Autodesk Inventor part; units mm, degrees
ref_plane "YZ Plane" through (0, 0, 0) normal (1, 0, 0) x (0, 1, 0)
ref_plane "XZ Plane" through (0, 0, 0) normal (0, 1, 0) x (-1, 0, 0)
ref_plane "XY Plane" through (0, 0, 0) normal (0, 0, 1) x (1, 0, 0)
sketch "Sketch1" plane through (0, 0, 0) normal (0, 0, 1) x (1, 0, 0)
  line L0 (0, 0) -> (50, 0)
  line L1 (50, 0) -> (140.0002, 119.9998)
  line L2 (140.0002, 119.9998) -> (141.8074, 169.9998)
  line L3 (172.7872, 168.8801) -> (170.5233, 106.2458)
  line L4 (0, -10) -> (50, -10)
  arc A0 (50, -10) -> (170.5233, 106.2458) centre (50, 110.602) ccw
  line L5 (0, -10) -> (0, 0)
  line L6 (141.8074, 169.9998) -> (172.7872, 168.8801)
  line L7 (140.0002, 119.9998) -> (171.0205, 119.9998)
  dimension "d0" = 150
  dimension "d1" = 126.87
  dimension "d2" = 50
  dimension "d3" = 145.2
  dimension "d4" = 31
  dimension "d5" = 10
  dimension "d6" = 50
extrude "Extrusion1" add sketch "Sketch1" along normal blind 25
sketch "Sketch2" plane through (0, -10, 0) normal (0, -1, 0) x (1, 0, 0)
  line L0 (0, 0) -> (50, 0)
  line L1 (50, 0) -> (50, 25)
  line L2 (0, 25) -> (50, 25)
  line L3 (0, 0) -> (0, 25)
  circle A0 centre (25, 12.5) radius 1.65
  point P0 (50, 12.5)
  point P1 (25, 25)
  dimension "d9" = 3.3
extrude "Extrusion2" cut sketch "Sketch2" against normal through all contours A0
sketch "Sketch3" plane through (172.7872, 168.8801, 25) normal (0.9993, -0.0361, 0) x (0, 0, -1)
  line L0 (25, -62.6752) -> (25, 0)
  line L1 (25, 0) -> (0, 0)
  line L2 (0, -62.6752) -> (0, 0)
  line L3 (25, -62.6752) -> (0, -62.6752)
  circle A0 centre (12.5, -22.6752) radius 2.15
  point P0 (25, -175.0111)
  point P1 (12.5, -62.6752)
  dimension "d12" = 4.3
  dimension "d13" = 40
extrude "Extrusion3" cut sketch "Sketch3" against normal through all contours A0
chamfer "Chamfer1" distance 10 angle 45 1 edges at (141.8074, 169.9998, 12.5)
properties part number "ESQUINA_REDONDEADA_TRASERA" material "Steel, Mild, Welded"
Input: part model. Units: mm. Frame: model coordinates. Give positions to 0.01 mm unless a question says otherwise; leave off trailing zeros. Order: outer loops, then holes, each group sorted by start corner. A loop starts at its lowest first (then second) coordinate and runs counter-clockwise, first axis right, second up. Notation, with made-up numbers: (-18, -3.5) - (18, -3.5) arc R23 cw to (18, 4.5) - close; hole circle Ø8 at (27.5, 77.5). An arc over 180 degrees is marked (long way). Put each result on its own line as item: value.
Item 1: Contact query for flat-ended pins moving along their axis: pin 1 (1.5 mm diameter, centred on x = 73, z = 21.5, fed in from -Y); pin 2 (2 mm diameter, centred on x = 79.5, z = 14.5, fed in from -Y); pin 3 (5.5 mm diameter, centred on x = 25, z = 12.5, fed in from +Y). Output: stop coordinate, or through.
Found:
pin 1: stops at y = -7.93
pin 2: stops at y = -6.58
pin 3: stops at y = 0
Item 2: Ray query, L1, parallel to Z at x = 25, y = -5; L2, parallel to Y at x = 16.5, z = 3.5; L3, parallel to X at y = 5, z = 11.5. Return the intervals inside material, ascending. Write a range as from..to.
Found:
L1: z = 0..10.85, 14.15..25
L2: y = -10..0
L3: x = 53.75..108.25
Item 3: Section query B-B, the plane y = 68.5. Return loops of the section in (x, z), then the cut area to 3 significant figures.
Found:
outline: (101.38, 0) - (163.01, 0) - (163.01, 25) - (101.38, 25) - close
area: 1,540 mm^2
Item 4: Section query C-C, the plane x = 87.5. Return loops of the section in (y, z), then the cut area to 3 significant figures.
Found:
outline: (-4.02, 0) - (50, 0) - (50, 25) - (-4.02, 25) - close
area: 1,350 mm^2
Item 5: Draft query along Y for faces 1 (the flat face through (124, 67, 25)), 2 (the cylindrical face through (156.665, 145.949, 10.514)), 3 (the flat face through (25, 0, 10)), 4 (the cylindrical face through (134.65, 24.7, 12.32)). Return one class per face: +Y half, -Y half, draft (parallel to the pull), parting line (faces both ways), or undercut.
Found:
face 1: draft
face 2: undercut
face 3: +Y half
face 4: -Y half
Item 6: Section query A-A, the plane z = 8. Return loops of the section in (x, y), then the cut area to 3 significant figures.
Found:
outline: (0, -10) - (50, -10) arc R120.6 ccw to (170.52, 106.25) - (172.79, 168.88) - (151.8, 169.64) - (141.45, 160.01) - (140, 120) - (50, 0) - (0, 0) - close
area: 9,140 mm^2
